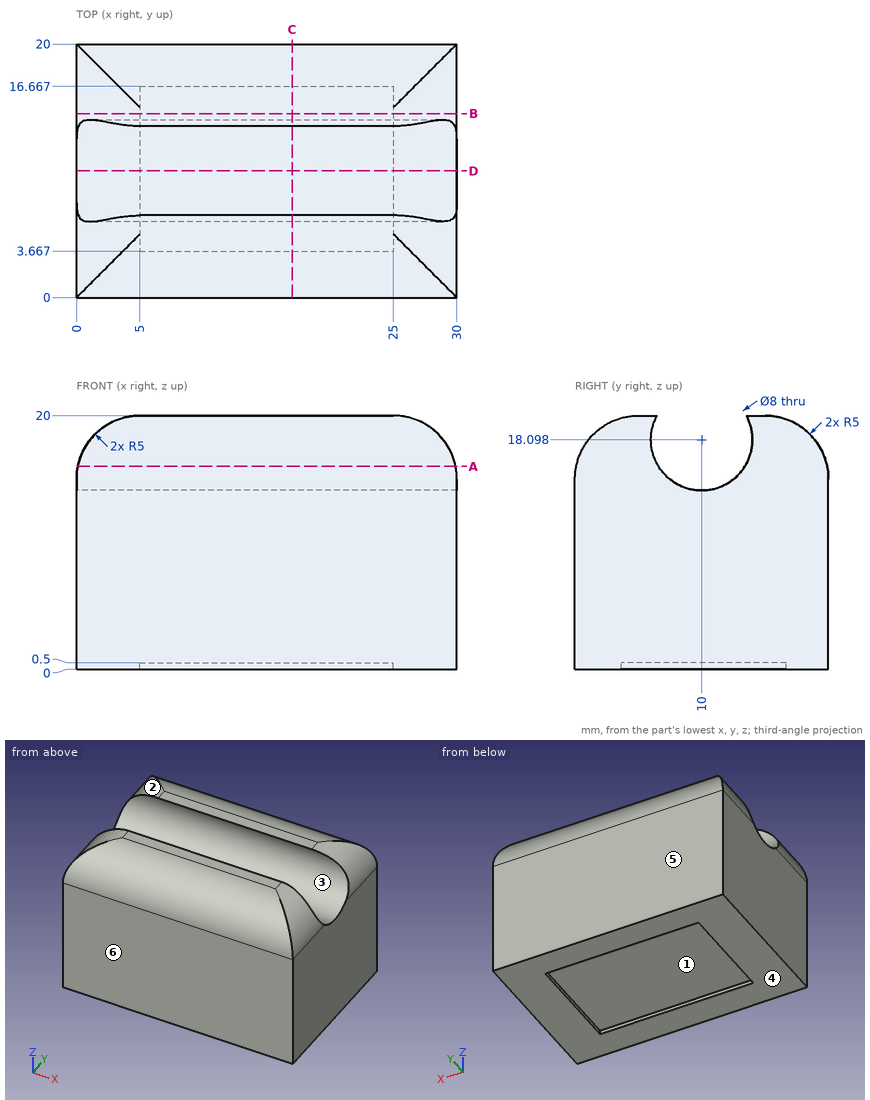
Check sheet for the drawn part. Datum: minimum x, y, z corner. Units: mm. A direction names the side the tool comes from. Round coordinates to 2 decimals unless told otherwise and drop trailing zeros. Order: outer loops, then holes, each group sorted by start corner. A loop starts at its lowest first (then second) coordinate and runs counter-clockwise, first axis right, second up. Notation, with made-up numbers: (-26.5, 3) - (17.5, 3) arc R12 cw to (17.5, 17) - close; hole circle Ø5 at (35.5, 17). An arc over 180 degrees is marked (long way). Use a Markdown table: item, result. Add a question column.
(1) Sectioned sample at B-B, the plane y = 14.5. Enter the section's corners in (x, z).
(2) Tool access check on the marked faces 1 and 2. Record the directions out of +Z, -Z, +X, -X, +Y, -Y that give a thin tool (end or side, any length) a straight path to the whole face; none if there is none.
(3) Sectioned sample at D-D, the plane y = 10. Enter the section's corners in (x, z), and give its area (3 significant figures).
(4) Depth check by flat-ended pin: pin 1 (6.5 mm diameter, centred on x = 12.5, y = 10.5, fed in from -Z). Enter the tip coordinate at first touch or a pass-through.
(5) Sectioned sample at C-C, the plane x = 17. Enter the section's corners in (y, z), and give its area (3 significant figures).
(6) Release check for a two-part mould opening along Y. For the marked faces 3, 4, 5 and 6 record: pulls with the +Y half, pulls with the -Y half, needs draft (parallel to the pull), parting line crosses it, or undercut.
(7) Material ranges on line 1 along Y through (x, z) = (15.5, 15.5) (1 decimal); line 2 along Y through (x, z) = (24.5, 19) (1 decimal); line 3 along Z through (x, y) = (20.5, 4.5) (1 decimal), recorded low to high. Write a range as [from, to].
(8) Sectioned sample at A-A, the plane z = 16. Enter the section's corners in (x, y), and give its area (3 significant figures).
Answers below:
| question | item | result |
|---|---|---|
| 1 | outline | (0, 0) - (5, 0) - (5, 0.5) - (25, 0.5) - (25, 0) - (30, 0) - (30, 15) arc R5 ccw to (25, 20) - (5, 20) arc R5 ccw to (0, 15) - close |
| 2 | face 1 | -Z |
| 2 | face 2 | +Z, -X, +Y, -Y |
| 3 | outline | (0, 0) - (5, 0) - (5, 0.5) - (25, 0.5) - (25, 0) - (30, 0) - (30, 14.1) - (0, 14.1) - close |
| 3 | area | 413 mm² |
| 4 | pin 1 | z = 0.5 |
| 5 | outline | (0, 0) - (3.67, 0) - (3.67, 0.5) - (16.67, 0.5) - (16.67, 0) - (20, 0) - (20, 15) arc R5 ccw to (15, 20) - (13.52, 20) arc R4 cw (long way) to (6.48, 20) - (5, 20) arc R5 ccw to (0, 15) - close |
| 5 | area | 343 mm² |
| 6 | face 3 | undercut |
| 6 | face 4 | needs draft |
| 6 | face 5 | pulls with the +Y half |
| 6 | face 6 | pulls with the -Y half |
| 7 | line 1 | [0, 7], [13, 20] |
| 7 | line 2 | [2, 6.1], [13.9, 18] |
| 7 | line 3 | [0.5, 20] |
| 8 | outline | (0.1, 0.1) - (29.9, 0.1) - (29.9, 6.59) - (0.1, 6.59) - close; (0.1, 13.41) - (29.9, 13.41) - (29.9, 19.9) - (0.1, 19.9) - close |
| 8 | area | 387 mm² |
